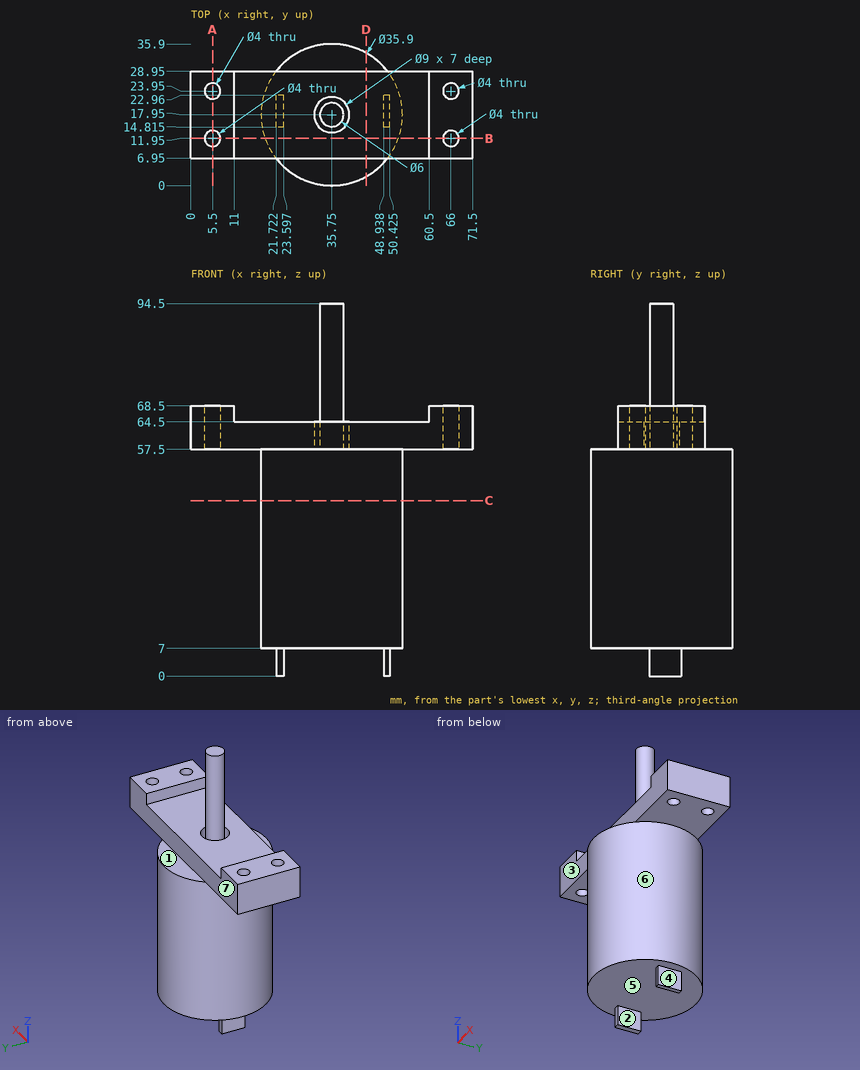
Print and shaded views of the part. All mm, measured from the part's lowest x, y and z. A direction names the side the tool comes from. Give positions to 0.01 mm unless a question says otherwise; leave off trailing zeros. Loops run counter-clockwise (first coordinate to the right, second up) from the corner with the lowest first, then second, coordinate; pieces in that order, holes last. Notation, with made-up numbers: (7, 22.25) - (17, 22.25) arc R12 ccw to (17, 35.25) - close; hole circle Ø11 at (73.5, -38.5). An arc over 180 degrees is marked (long way). One line per item, written item: value. Start each with the question number.
1. Slice it at D-D (x = 44.5). List the corners of the cut face in (y, z).
2. Slice it at A-A (x = 5.5). List the corners of the cut face in (y, z), plus the area to 3 significant figures.
3. Which spindle directions (+Z, -Z, +X, -X, +Y, -Y) get a long thin tool onto all of the face, cutting with end or side? Do the marked faces 1, 2, 3 and 4. Say none if no direction does.
4. Pin check, flat tips, straight feed: pin 1 (12 mm diameter, centred on x = 39, y = 24, fed in from -Z); pin 2 (9 mm diameter, centred on x = 30, z = 65, fed in from +Y); pin 3 (4.5 mm diameter, centred on x = 66, y = 23.95, fed in from -Z). Stop position of each tip, or through.
5. Slice it at C-C (z = 44.5). List the corners of the cut face in (x, y).
6. Pull direction X, two halves, no side cores. Call the marked faces 5, 6 and 7: pulls with the +X half, pulls with the -X half, needs draft (parallel to the pull), parting line crosses it, or undercut.
7. Probe L1, parallel to Y at x = 35.75, z = 61.75; L2, parallel to Y at x = 66, z = 65.25; L3, parallel to X at y = 11.5, z = 61. List the from-to ranges inside material, lowest first. Write a range as from..to.
8. Slice it at B-B (y = 11.95). List the corners of the cut face in (x, z).
Solution:
1. outline: (2.28, 7) - (33.62, 7) - (33.62, 57.5) - (28.95, 57.5) - (28.95, 64.5) - (6.95, 64.5) - (6.95, 57.5) - (2.28, 57.5) - close
2. outline: (6.95, 57.5) - (9.95, 57.5) - (9.95, 68.5) - (6.95, 68.5) - close; (13.95, 57.5) - (21.95, 57.5) - (21.95, 68.5) - (13.95, 68.5) - close; (25.95, 57.5) - (28.95, 57.5) - (28.95, 68.5) - (25.95, 68.5) - close
2. area: 154 mm^2
3. face 1: +Z, +X, -X, +Y
3. face 2: -Z, +Y, -Y
3. face 3: +Z, +X, -X, -Y
3. face 4: -Z, +X, +Y, -Y
4. pin 1: stops at z = 7
4. pin 2: stops at y = 28.95
4. pin 3: stops at z = 57.5
5. outline: circle Ø35.9 at (35.75, 17.95)
6. face 5: undercut
6. face 6: parting line crosses it
6. face 7: needs draft
7. L1: y = 6.95..13.45, 14.95..20.95, 22.45..28.95
7. L2: y = 6.95..9.95, 13.95..21.95, 25.95..28.95
7. L3: x = 0..3.55, 7.45..64.05, 67.95..71.5
8. outline: (0, 57.5) - (3.5, 57.5) - (3.5, 68.5) - (0, 68.5) - close; (7.5, 57.5) - (18.83, 57.5) - (18.83, 7) - (52.67, 7) - (52.67, 57.5) - (64, 57.5) - (64, 68.5) - (60.5, 68.5) - (60.5, 64.5) - (11, 64.5) - (11, 68.5) - (7.5, 68.5) - close; (68, 57.5) - (71.5, 57.5) - (71.5, 68.5) - (68, 68.5) - close
